Source: CAD feature listing. Evaluate the final solid. Frame: model axes, mm. A direction names the side the tool comes from. Give positions to 0.01 mm unless a question says otherwise; leave off trailing zeros. Loops run counter-clockwise (first coordinate to the right, second up) from the corner with the lowest first, then second, coordinate; pieces in that order, holes last. Notation, with made-up numbers: (22.25, -1.75) - (54.25, -1.75) arc R16 cw to (54.25, 6.25) - close; hole circle Ø6 at (5.5, -6). An arc over 180 degrees is marked (long way). Put each result on its own line as item: value.
```python
from build123d import *

# Parameters (mm, degrees)
SKETCH1_R             = 32.5
SKETCH1_R_2           = 30.5
BOSS_EXTRUDE1_DEPTH   = 3.5
SKETCH1_R_3           = 27
SKETCH1_R_4           = 25
BOSS_EXTRUDE1_2_DEPTH = 3.5
SKETCH1_3_R           = 30.5
SKETCH1_3_R_2         = 27
BOSS_EXTRUDE2_DEPTH   = 3.4


with BuildPart() as part:
    # Sketch1 → Boss-Extrude1 (new, symmetric)
    with BuildSketch(Plane(origin=(0, 0, 0), x_dir=(1, 0, 0), z_dir=(0, 1, 0))):
        Circle(SKETCH1_R)
        Circle(SKETCH1_R_2, mode=Mode.SUBTRACT)
    extrude(amount=BOSS_EXTRUDE1_DEPTH, both=True)



with BuildPart() as body_2:
    # Sketch1 → Boss-Extrude1 2 (new, symmetric)
    with BuildSketch(Plane(origin=(0, 0, 0), x_dir=(1, 0, 0), z_dir=(0, 1, 0))):
        Circle(SKETCH1_R_3)
        Circle(SKETCH1_R_4, mode=Mode.SUBTRACT)
    extrude(amount=BOSS_EXTRUDE1_2_DEPTH, both=True)


with BuildPart() as part_1:
    add(part.part)

    add(body_2.part)  # Boss-Extrude2 merges body 2
    # Sketch1<3> → Boss-Extrude2 (add, symmetric)
    with BuildSketch(Plane(origin=(0, 0, 0), x_dir=(1, 0, 0), z_dir=(0, 1, 0))):
        Circle(SKETCH1_3_R)
        Circle(SKETCH1_3_R_2, mode=Mode.SUBTRACT)
    extrude(amount=BOSS_EXTRUDE2_DEPTH, both=True)


solid = part_1.part
```
1) Material intervals for line 1 along Z through (x, y) = (0, -3.45); line 2 along Z through (x, y) = (0.5, 2) (3 decimals); line 3 along X through (y, z) = (-2.75, 17.5), sorted ascending. Write a range as [from, to].
Check result:
line 1: [-32.5, -30.5], [-27, -25], [25, 27], [30.5, 32.5]
line 2: [-32.496, -24.995], [24.995, 32.496]
line 3: [-27.39, -17.85], [17.85, 27.39]
2) Section query C-C, the plane y = -2.5. Output: boundary loops of the cut face in (x, z), plus the area to 3 significant figures.
Check result:
outline: circle Ø65 at (0, 0); hole circle Ø50 at (0, 0)
area: 1,350 mm²
3) Access query for faces 1 (the flat face through (11, 3.4, 25)), 2 (the flat face through (-10, 3.5, -29)). Directions: +Z, -Z, +X, -X, +Y, -Y. A direction counts if a zero-diameter tool reaches every point of the face in a straight line with its end or side. Return the directions, or none.
Check result:
face 1: +Y
face 2: +Z, -Z, +X, -X, +Y
4) Section query B-B, the plane z = 0. Output: boundary loops of the cut face in (x, y), plus the area to 3 significant figures.
Check result:
outline: (-32.5, -3.5) - (-30.5, -3.5) - (-30.5, -3.4) - (-27, -3.4) - (-27, -3.5) - (-25, -3.5) - (-25, 3.5) - (-27, 3.5) - (-27, 3.4) - (-30.5, 3.4) - (-30.5, 3.5) - (-32.5, 3.5) - close; (25, -3.5) - (27, -3.5) - (27, -3.4) - (30.5, -3.4) - (30.5, -3.5) - (32.5, -3.5) - (32.5, 3.5) - (30.5, 3.5) - (30.5, 3.4) - (27, 3.4) - (27, 3.5) - (25, 3.5) - close
area: 104 mm²
5) Section query D-D, the plane x = 26. Output: boundary loops of the cut face in (y, z).
Check result:
outline: (-3.5, -19.5) - (3.5, -19.5) - (3.5, -15.95) - (3.4, -15.95) - (3.4, -7.28) - (3.5, -7.28) - (3.5, 7.28) - (3.4, 7.28) - (3.4, 15.95) - (3.5, 15.95) - (3.5, 19.5) - (-3.5, 19.5) - (-3.5, 15.95) - (-3.4, 15.95) - (-3.4, 7.28) - (-3.5, 7.28) - (-3.5, -7.28) - (-3.4, -7.28) - (-3.4, -15.95) - (-3.5, -15.95) - close
6) Section query A-A, the plane x = 0. Output: boundary loops of the cut face in (y, z).
Check result:
outline: (-3.5, -32.5) - (3.5, -32.5) - (3.5, -30.5) - (3.4, -30.5) - (3.4, -27) - (3.5, -27) - (3.5, -25) - (-3.5, -25) - (-3.5, -27) - (-3.4, -27) - (-3.4, -30.5) - (-3.5, -30.5) - close; (-3.5, 25) - (3.5, 25) - (3.5, 27) - (3.4, 27) - (3.4, 30.5) - (3.5, 30.5) - (3.5, 32.5) - (-3.5, 32.5) - (-3.5, 30.5) - (-3.4, 30.5) - (-3.4, 27) - (-3.5, 27) - close
7) Mould query, pull axis Z, two halves, no side actions, for faces 3 (the flat face through (-10, -3.5, -29)), 4 (the cylindrical face through (31, 0.05, -9.76)), 5 (the flat face through (11, -3.4, 25)). Classes: pulls with the +Z half, pulls with the -Z half, needs draft (parallel to the pull), parting line crosses it, or undercut.
Check result:
face 3: needs draft
face 4: parting line crosses it
face 5: undercut
8) Pin query (flat end, axial travel): P1, Ø2, axis at y = -2.5, z = 4, coming from the +X side; P2, Ø1.5, axis at x = 3.5, y = -2.5, coming from the -Z side; P3, Ø3, axis at y = 1.5, z = 12, coming from the +X side. Return the tip coordinate at first contact, or that it passes through.
Check result:
P1: x = 32.36
P2: z = -32.38
P3: x = 30.76
